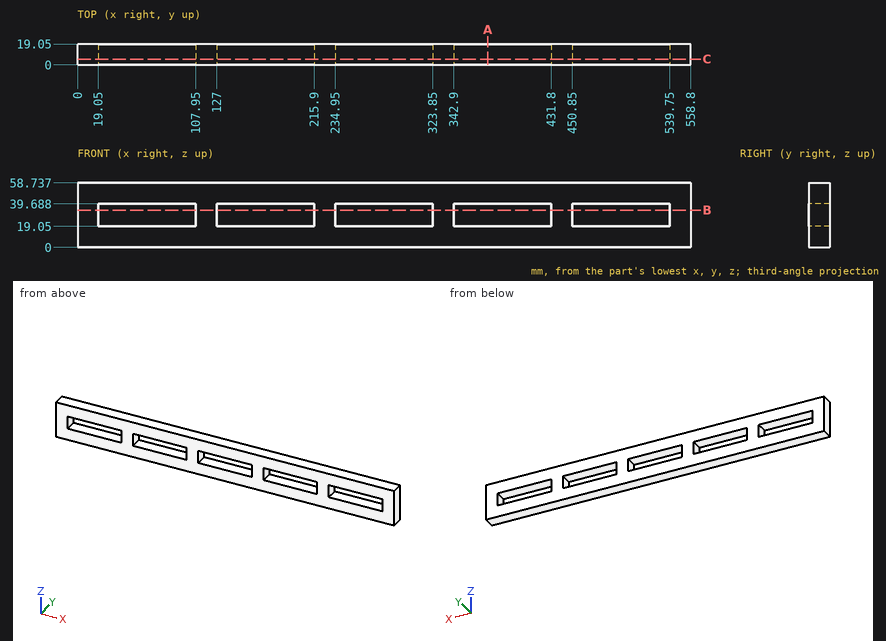
Verification items for this drawing (mm, ordinates from the low corner). Give positions to 0.01 mm unless a question says otherwise; leave off trailing zeros. Loops run counter-clockwise (first coordinate to the right, second up) from the corner with the lowest first, then second, coordinate; pieces in that order, holes last.
(1) Thickness scan on L1, parallel to X at y = 14, z = 33; L2, parallel to Z at x = 287, y = 11.5. Record the ranges inside material, lowest first.
From the geometry:
L1: x = 0 to 19.05, 107.95 to 127, 215.9 to 234.95, 323.85 to 342.9, 431.8 to 450.85, 539.75 to 558.8
L2: z = 0 to 19.05, 39.69 to 58.74
(2) Section check B-B on z = 34. Record the cut outline in (x, y).
From the geometry:
outline: (0, 0) - (19.05, 0) - (19.05, 19.05) - (0, 19.05) - close; (107.95, 0) - (127, 0) - (127, 19.05) - (107.95, 19.05) - close; (215.9, 0) - (234.95, 0) - (234.95, 19.05) - (215.9, 19.05) - close; (323.85, 0) - (342.9, 0) - (342.9, 19.05) - (323.85, 19.05) - close; (431.8, 0) - (450.85, 0) - (450.85, 19.05) - (431.8, 19.05) - close; (539.75, 0) - (558.8, 0) - (558.8, 19.05) - (539.75, 19.05) - close
(3) Section check A-A on x = 374. Record the cut outline in (y, z).
From the geometry:
outline: (0, 0) - (19.05, 0) - (19.05, 19.05) - (0, 19.05) - close; (0, 39.69) - (19.05, 39.69) - (19.05, 58.74) - (0, 58.74) - close
(4) Section check C-C on y = 5.25. Record the cut outline in (x, z), then the cut area to 4 significant figures.
From the geometry:
outline: (0, 0) - (558.8, 0) - (558.8, 58.74) - (0, 58.74) - close; hole (19.05, 19.05) - (107.95, 19.05) - (107.95, 39.69) - (19.05, 39.69) - close; hole (127, 19.05) - (215.9, 19.05) - (215.9, 39.69) - (127, 39.69) - close; hole (234.95, 19.05) - (323.85, 19.05) - (323.85, 39.69) - (234.95, 39.69) - close; hole (342.9, 19.05) - (431.8, 19.05) - (431.8, 39.69) - (342.9, 39.69) - close; hole (450.85, 19.05) - (539.75, 19.05) - (539.75, 39.69) - (450.85, 39.69) - close
area: 23,650 mm2
